Input: part model. Units: mm. Frame: model coordinates. Face numbers are marked on the shaded views. A direction names the side the tool comes from. Coordinates: 2 decimals unless noted, no trailing zeros. Write each loop counter-clockwise with the first axis right and the second up, starting at its lowest first coordinate (ties: lowest second). Pieces come first, ordered by that corner, then holes. Notation, with made-up numbers: M 37,44 L 45,44 A16 ccw 45,59 Z; hole C 69.25,-19 d8. An arc over 180 degrees is marked long. Use one line per item in the form item = value.
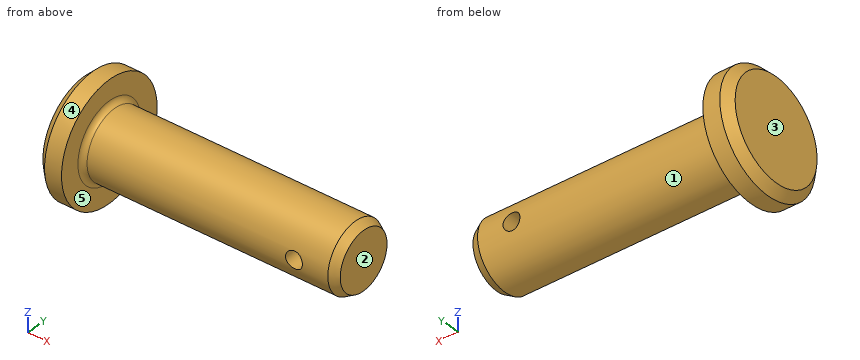
from build123d import *

# Parameters (mm, degrees)
VERRUNDUNG1_R                               = 0.6
SCHNITT_LINEAR_AUSTRAGEN1_REACH             = 9
SKIZZE2_R                                   = 1
SCHNITT_LINEAR_AUSTRAGEN1_DIRECTION_2_REACH = 9


with BuildPart() as part:
    # Skizze1 → Rotation1 (revolve)
    with BuildSketch(Plane.XY):
        Polygon((-3, 0), (-3, 6), (-2, 7), (0, 7), (0, 4), (29, 4), (30, 3.422649731), (30, 0), align=None)
    revolve(axis=Axis((30, 0, 0), (-1, 0, 0)))

    # Verrundung1
    verrundung1_edges = [part.edges().sort_by_distance(p)[0] for p in [
        (0, -4, 0),
    ]]
    fillet(verrundung1_edges, radius=VERRUNDUNG1_R)

    # Skizze2 → Schnitt-Linear austragen1 (cut, up to next)
    with BuildSketch(Plane(origin=(0, 0, 0), x_dir=(1, 0, 0), z_dir=(0, 1, 0)), mode=Mode.PRIVATE) as schnitt_linear_austragen1_sk1:
        with Locations((25, 0)):
            Circle(SKIZZE2_R)
    schnitt_linear_austragen1_tool1 = extrude(schnitt_linear_austragen1_sk1.sketch, amount=-SCHNITT_LINEAR_AUSTRAGEN1_REACH, mode=Mode.PRIVATE) & part.part
    add(schnitt_linear_austragen1_tool1.solids().sort_by_distance((25, 0, 0))[0], mode=Mode.SUBTRACT)

    # Skizze2 → Schnitt-Linear austragen1 direction 2 (cut, up to next)
    with BuildSketch(Plane(origin=(0, 0, 0), x_dir=(1, 0, 0), z_dir=(0, 1, 0)), mode=Mode.PRIVATE) as schnitt_linear_austragen1_direction_2_sk1:
        with Locations((25, 0)):
            Circle(SKIZZE2_R)
    schnitt_linear_austragen1_direction_2_tool1 = extrude(schnitt_linear_austragen1_direction_2_sk1.sketch, amount=SCHNITT_LINEAR_AUSTRAGEN1_DIRECTION_2_REACH, mode=Mode.PRIVATE) & part.part
    add(schnitt_linear_austragen1_direction_2_tool1.solids().sort_by_distance((25, 0, 0))[0], mode=Mode.SUBTRACT)


solid = part.part
(1) Section query B-B on x = 21. Return the cut outline in (y, z).
Computed:
outline = C 0,0 d8
(2) Set-up query: the marked faces 1 and 2. Return all of +Z, -Z, +X, -X, +Y, -Y with unobstructed straight access to the full face (end or side cutting, diameter ignored); none if empty.
Computed:
face_1 = +X
face_2 = +Z, -Z, +X, +Y, -Y
(3) First-contact query: pin 1 Ø4 at (x, z) = (14.5, -1.5) entering from -Y; pin 2 Ø2 at (x, y) = (5, -2) entering from +Z; pin 3 Ø1.6 at (x, z) = (25, 0) entering from -Y. Flat tips, straight axial feed; report the tip coordinate or a pass-through.
Computed:
pin_1 = -4
pin_2 = 3.87
pin_3 = through
(4) Section query C-C on x = 25. Return the cut outline in (y, z).
Computed:
outline = M -3.87,-1 A4 ccw 3.87,-1 Z; M -3.87,1 L 3.87,1 A4 ccw Z
(5) Section query A-A on z = 0. Return the cut outline in (x, y).
Computed:
outline = M -3,-6 L -2,-7 L 0,-7 L 0,-4.6 A0.6 cw 0.6,-4 L 24,-4 L 24,4 L 0.6,4 A0.6 cw 0,4.6 L 0,7 L -2,7 L -3,6 Z; M 26,-4 L 29,-4 L 30,-3.42 L 30,3.42 L 29,4 L 26,4 Z
(6) Pull-direction query (X, two-part tool) for the marked faces 3, 4 and 5; classes: pulls with the +X half, pulls with the -X half, needs draft (parallel to the pull), parting line crosses it, or undercut.
Computed:
face_3 = pulls with the -X half
face_4 = needs draft
face_5 = pulls with the +X half
(7) Line query: probe 1 along X at (y, z) = (-1.9, 0); probe 2 along X at (y, z) = (-2.5, 4.75); probe 3 along X at (y, z) = (-0.5, 0.5). Output: solid intervals per line, ascending.
Computed:
probe_1 = -3 to 24, 26 to 30
probe_2 = -3 to 0
probe_3 = -3 to 24.13, 25.87 to 30
